Part print with two shaded views. Sizes in mm from the minimum x, y, z corner. A direction names the side the tool comes from. Give positions to 0.01 mm unless a question says otherwise; leave off trailing zeros. Write each loop counter-clockwise with the first axis right and the second up, starting at its lowest first coordinate (ties: lowest second). Pieces come first, ordered by that corner, then holes. Notation, with made-up numbers: (-8, 79) -> (3, 79) arc R19 ccw to (3, 112) -> close; hole circle Ø5 at (11.5, -27). An arc over 180 degrees is marked (long way). Answer as a JSON object with one key per item and string values.
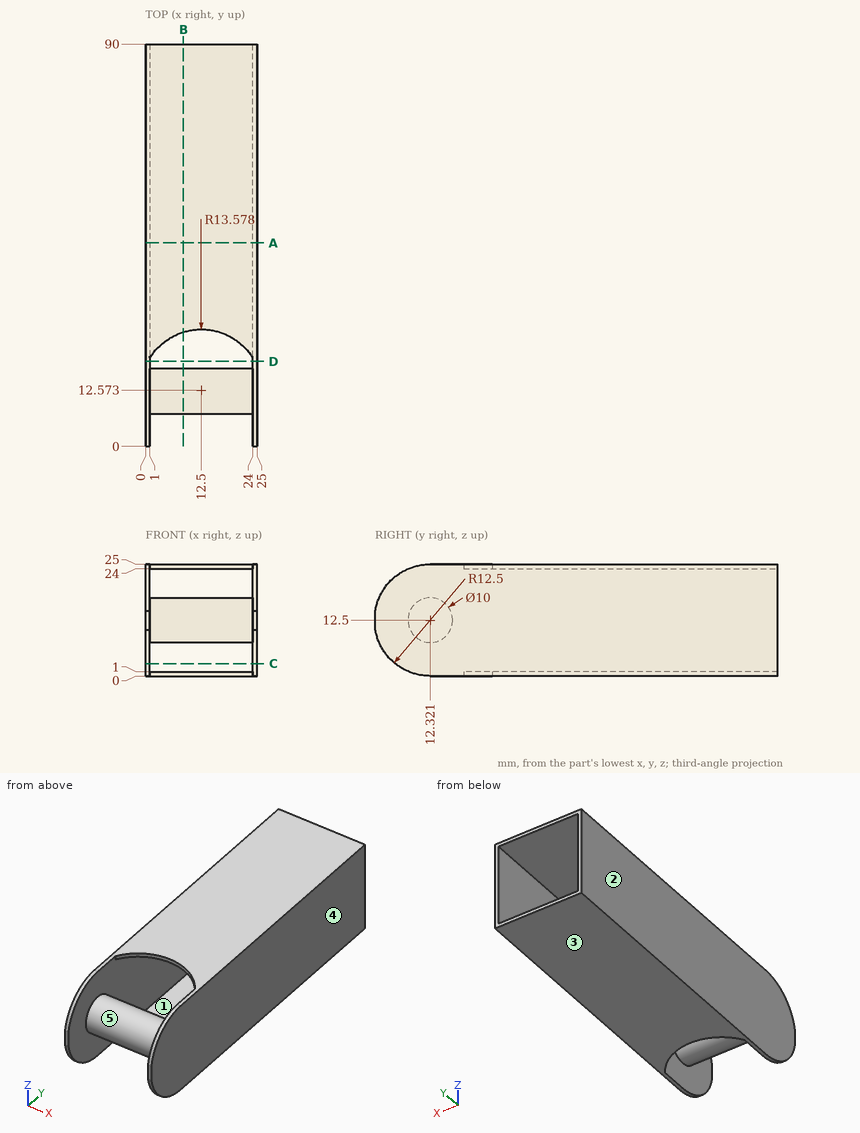
1) Mould opens along X. For the marked faces 3, 4 and 5 say: released by +X, released by -X, zero draft, split by the parting line, or undercut.
Model answer:
{"face 3": "zero draft", "face 4": "released by +X", "face 5": "undercut"}
2) Wall check: probe 1 along X at (y, z) = (36.5, 19.5); probe 2 along Z at (x, y) = (5.5, 9.5). Give the ranges that are in metal, low to high.
Model answer:
{"probe 1": "x = 0 to 1, 24 to 25", "probe 2": "z = 8.37 to 16.63"}
3) 3-axis set-ups, long thin cutter, end or side, ignore diameter. For the marked faces 1 and 2: which of +Z, -Z, +X, -X, +Y, -Y reach the whole face in a straight line?
Model answer:
{"face 1": "+Y, -Y", "face 2": "+Z, -Z, -X, +Y, -Y"}
4) Slice it at B-B (x = 8.5). List the corners of the cut face in (y, z).
Model answer:
{"outline": "circle Ø10 at (12.32, 12.5); (25.55, 0) -> (90, 0) -> (90, 1) -> (25.55, 1) -> close; (25.55, 24) -> (90, 24) -> (90, 25) -> (25.55, 25) -> close"}
5) Pin check, flat tips, straight feed: pin 1 (2 mm diameter, centred on y = 10, z = 22, fed in from -X); pin 2 (4 mm diameter, centred on x = 13, z = 9, fed in from +Y); pin 3 (12 mm diameter, centred on x = 13, y = 18, fed in from -Z); pin 4 (10 mm diameter, centred on x = 10.5, z = 13.5, fed in from -Y). Stop position of each tip, or through.
Model answer:
{"pin 1": "stops at x = 0", "pin 2": "stops at y = 17.09", "pin 3": "stops at z = 7.5", "pin 4": "stops at y = 7.32"}
6) Slice it at C-C (z = 2.75). List the corners of the cut face in (x, y).
Model answer:
{"outline": "(0, 4.5) -> (1, 4.5) -> (1, 90) -> (0, 90) -> close; (24, 4.5) -> (25, 4.5) -> (25, 90) -> (24, 90) -> close"}
7) Slice it at D-D (y = 19). List the corners of the cut face in (x, z).
Model answer:
{"outline": "(0, 0) -> (1, 0) -> (1, 25) -> (0, 25) -> close; (24, 0) -> (25, 0) -> (25, 25) -> (24, 25) -> close"}
8) Slice it at A-A (y = 45.5). List the corners of the cut face in (x, z).
Model answer:
{"outline": "(0, 0) -> (25, 0) -> (25, 25) -> (0, 25) -> close; hole (1, 1) -> (24, 1) -> (24, 24) -> (1, 24) -> close"}
